Autodesk Fusion 360 part; units mm, degrees
sketch "Sketch1" plane through (0, 0, 0) normal (0, 0, 1) x (1, 0, 0)
  line L0 (0, 0) -> (0, 80)
  line L1 (0, 80) -> (80, 80)
  line L2 (8, 6) -> (8, 68)
  line L3 (12, 72) -> (74, 72)
  line L4 (80, 78) -> (80, 80)
  line L5 (0, 0) -> (2, 0)
  arc A0 (74, 72) -> (80, 78) centre (74, 78) ccw
  arc A1 (2, 0) -> (8, 6) centre (2, 6) ccw
  arc A2 (12, 72) -> (8, 68) centre (12, 68) ccw
  dimension "d1" = 80
  dimension "d2" = 80
  dimension "d4" = 6
  dimension "d5" = 6
  dimension "d6" = 4
extrude "Extrude1" add sketch "Sketch1" along normal mid plane 1450
sketch "Sketch4" plane through (0, 0, 0) normal (-1, 0, 0) x (0, 0, 1)
  line L0 (-725, 0) -> (725, 0) construction
  line L1 (725, 0) -> (725, 80) construction
  line L2 (725, 80) -> (-725, 80) construction
  line L3 (-725, 80) -> (-725, 0) construction
  line L4 (-725, 0) -> (725, 0) construction
  line L5 (-725, 80) -> (725, 80) construction
  line L6 (-725, 0) -> (-725, 80) construction
  line L7 (725, 80) -> (725, 0) construction
  line L8 (0, 0) -> (0, 80) construction
  line L9 (-725, 40) -> (725, 40) construction
  line L10 (-725, 80) -> (-725, -420) construction
  line L11 (285, 80) -> (285, -420) construction
  line L12 (365, 80) -> (365, -420) construction
  line L13 (425, 80) -> (425, -420) construction
  line L14 (620, 80) -> (620, -420) construction
  line L15 (690, 80) -> (690, -420) construction
  line L16 (629, 31) -> (681, 31)
  arc A0 (681, 31) -> (681, 49) centre (681, 40) ccw
  line L17 (681, 49) -> (629, 49)
  arc A1 (629, 49) -> (629, 31) centre (629, 40) ccw
  line L18 (620, 40) -> (690, 40) construction
  circle A2 centre (285, 40) radius 9
  circle A3 centre (365, 40) radius 9
  circle A4 centre (425, 40) radius 9
  dimension "d16" = 1010
  dimension "d17" = 1090
  dimension "d18" = 1150
  dimension "d19" = 1345
  dimension "d20" = 1415
  dimension "d21" = 18
  dimension "d22" = 18
  dimension "d23" = 18
  dimension "d24" = 18
extrude "Extrude4" cut sketch "Sketch4" against normal through all
sketch "Sketch5" plane through (0, 80, 0) normal (0, 1, 0) x (-1, 0, 0)
  line L0 (0, -725) -> (0, 725) construction
  line L1 (0, 725) -> (-80, 725)
  line L2 (-80, 725) -> (-80, -725) construction
  line L3 (-80, -725) -> (0, -725) construction
  line L4 (-80, -725) -> (-80, 725) construction
  line L5 (0, -725) -> (-80, -725) construction
  line L6 (0, -725) -> (0, 725) construction
  line L7 (-30, -725) -> (-30, 725) construction
  line L8 (-80, -725) -> (384.3429, -725) construction
  line L9 (-80, -695) -> (384.3429, -695) construction
  line L10 (-80, -555) -> (384.3429, -555) construction
  line L11 (-80, -155) -> (384.3429, -155) construction
  circle A0 centre (-30, -695) radius 9
  circle A1 centre (-30, -555) radius 9
  circle A2 centre (-30, -155) radius 8
  dimension "d26" = 30
  dimension "d27" = 30
  dimension "d28" = 170
  dimension "d29" = 570
  dimension "d30" = 18
  dimension "d31" = 18
  dimension "d32" = 16
extrude "Extrude5" cut sketch "Sketch5" against normal through all
ref_plane "WorkPlane1" through (40, 74, 0) normal (0, 1, 0) x (-1, 0, 0)
sketch "Sketch6" plane through (40, 74, 0) normal (0, 1, 0) x (1, 0, 0)
  line L0 (-40, 725) -> (-40, -725) construction
  line L1 (-40, 725) -> (40, 725) construction
  line L2 (40, 725) -> (40, -725) construction
  line L3 (40, 725) -> (-288.3779, 725)
  line L4 (40, 355) -> (-288.3779, 355)
  line L5 (-43.5, 725) -> (-43.5, -725) construction
  circle A0 centre (-43.5, 355) radius 8
  dimension "d35" = 370
  dimension "d36" = 3.5
  dimension "d37" = 16
extrude "Extrude6" add sketch "Sketch6" against normal blind 284
ref_plane "WorkPlane2" through (-3.5, -200, -355) normal (0, -1, 0) x (-1, 0, 0)
sketch "Sketch7" plane through (-3.5, -200, -355) normal (0, -1, 0) x (1, 0, 0)
  circle A0 centre (0, 0) radius 16
  dimension "d41" = 32
extrude "Extrude7" add sketch "Sketch7" against normal blind 5
chamfer "Chamfer1" distance 1 angle 45 1 edges at (-10.9586, -210, -357.8929)
The listing builds one solid part. Answer for the finished solid, in the listing's coordinates (mm). A direction names the side the tool comes from. Coordinates: 2 decimals unless noted, no trailing zeros. Write each loop counter-clockwise with the first axis right and the second up, starting at its lowest first coordinate (ties: lowest second). Pieces come first, ordered by that corner, then holes. Notation, with made-up numbers: M 80,18.5 L 109,18.5 A28 ccw 109,39.5 Z; hole C 72.5,19 d1. An arc over 180 degrees is marked long. Put each result on its own line as item: value. Start each with the question number.
1. A cutting plane is placed at A-A on z = -1. Write down the section's boundary in (x, y).
2. Flat-ended cylindrical pins translate along their axes: P1, Ø1.6, axis at x = 1, z = 26.5, coming from the -Y side; P2, Ø24, axis at y = 44, z = -132, coming from the -X side; P3, Ø21, axis at x = 30, z = -155, coming from the -Y side; P4, Ø20.5, axis at x = 30, z = -555, coming from the +Y side. Find the tip coordinate at first contact, or state that the pin passes through.
3. A cutting plane is placed at B-B on x = 54. Write down the section's boundary in (y, z).
4. Which of the six approach directions +Z, -Z, +X, -X, +Y, -Y give full straight-line access (tool end or side, diameter ignored) to faces 1 (the cylindrical face through (-6.97, -197.54, -370.62)), 2 (the flat face through (-11, -195, -351)), 3 (the flat face through (22, 73, 725))?
5. Consider line 1 (X direction, y = 76.5, z = -555); line 2 (X direction, y = 15, z = -174); line 3 (X direction, y = 76, z = -555). Determine where each line is inside the solid, lowest interval first. Write a range as from..to.
6. A cutting plane is placed at C-C on y = -42. Write down the section's boundary in (x, z).
Resolved:
1. outline: M 0,0 L 2,0 A6 ccw 8,6 L 8,68 A4 cw 12,72 L 74,72 A6 ccw 80,78 L 80,80 L 0,80 Z
2. P1: stops at y = 0
2. P2: stops at x = 0
2. P3: stops at y = 72
2. P4: stops at y = 80
3. outline: M 72,-725 L 80,-725 L 80,725 L 72,725 Z
4. face 1: -Y
4. face 2: none
4. face 3: +Z, +X, -X, +Y, -Y
5. line 1: x = 0..21, 39..79.81
5. line 2: x = 0..8
5. line 3: x = 0..21, 39..79.66
6. outline: C -3.5,-355 d16
